```python
from build123d import *

# Parameters (mm, degrees)
F0_R     = 15.054767
F0_R_2   = 12.024096
F1_DEPTH = 100
F2_R     = 14.954944
F2_R_2   = 9.478125
F3_DEPTH = 15.1
F4_DEPTH = 88.3


with BuildPart() as f1:
    # F0 (on Front) → F1 (new body)
    with BuildSketch(Plane.XZ):
        Circle(F0_R)
        Circle(F0_R_2, mode=Mode.SUBTRACT)
    extrude(amount=F1_DEPTH)

    # F2 (on Right) → F3 (join)
    with BuildSketch(Plane.YZ):
        Circle(F2_R)
        Circle(F2_R_2, mode=Mode.SUBTRACT)
    extrude(amount=F3_DEPTH)

    # F2 (on Right) → F4 (join)
    with BuildSketch(Plane.YZ):
        Circle(F2_R)
        Circle(F2_R_2, mode=Mode.SUBTRACT)
    extrude(amount=-F4_DEPTH)


solid = f1.part
```
CAD build for the part. Positions are in the model's coordinates, mm. A direction names the side the tool comes from. Round coordinates to 2 decimals unless told otherwise and drop trailing zeros. Loops run counter-clockwise (first coordinate to the right, second up) from the corner with the lowest first, then second, coordinate; pieces in that order, holes last. Notation, with made-up numbers: M -34,41.25 L 9,41.25 A34 ccw 9,71.25 Z; hole C 44.5,54 d2. An arc over 180 degrees is marked long. Return JSON: item names as keys, results as strings. Group by question number.
(1) Saw through at B-B, the plane x = 9. List the corners of the cut face in (y, z), and give its area (3 significant figures).
(2) Saw through at C-C, the plane y = -90. List the corners of the cut face in (x, z).
(3) Mould opens along Y. For faces 1 (the cylindrical face through (15.054, -3.62, -0.144)), 2 (the flat face through (-10, -100, -7)), 3 (the cylindrical face through (-15.04, -49.3, 0.66)) say: +Y half, -Y half, draft (parallel to the pull), parting line (faces both ways), or undercut.
(4) Wall check: probe 1 along Y at (x, z) = (-22, 0); probe 2 along X at (y, z) = (-45, 0). Give the ranges that are in metal, low to high. Write a range as [from, to].
(5) Tool access for faces 4 (the cylindrical face through (-12.012, -53.808, 0.529)), 5 (the flat face through (15.1, 0, -10)), 6 (the cylindrical face through (12.023, -3.62, -0.153)), 7 (the flat face through (-88.3, 0, -10)), 8 (the flat face through (-13, 0, 0)): list every direction of +Z, -Z, +X, -X, +Y, -Y with a clear straight run to the whole face (end or side of a thin tool).
(6) Saw through at D-D, the plane x = -41.5. List the corners of the cut face in (y, z).
(7) Saw through at A-A, the plane z = 0. List the corners of the cut face in (x, y).
(8) Drop flat-ended pins along their axis: P1, Ø12, axis at x = -44, y = -4.5, coming from the +Z side; P2, Ø5, axis at y = -27.5, z = 4, coming from the +X side; P3, Ø2.5, axis at x = -12, z = 1, coming from the +Y side; P4, Ø8, axis at x = 3.5, z = 10, coming from the +Y side. Give the stop position or say it passes through.
Answer list:
{
 "1": {"outline": "M -100,-12.07 L -8.83,-12.07 A14.95 ccw long -8.83,12.07 L -100,12.07 L -100,7.97 L -12.65,7.97 A14.95 ccw -12.65,-7.97 L -100,-7.97 Z; hole M -5.12,-7.97 L 0,-7.97 L 0,-9.48 A9.48 ccw 0,9.48 L 0,7.97 L -5.12,7.97 A9.48 ccw Z", "area": "1,160 mm2"},
 "2": {"outline": "C 0,0 d30.11; hole C 0,0 d24.05"},
 "3": {"face 1": "undercut", "face 2": "-Y half", "face 3": "draft"},
 "4": {"probe 1": "[-14.95, -9.48], [9.48, 14.95]", "probe 2": "[-15.05, -12.02], [12.02, 15.05]"},
 "5": {"face 4": "-Y", "face 5": "+Z, -Z, +X, +Y, -Y", "face 6": "none", "face 7": "+Z, -Z, -X, +Y, -Y", "face 8": "+X, -X"},
 "6": {"outline": "C 0,0 d29.91; hole C 0,0 d18.96"},
 "7": {"outline": "M -88.3,-14.95 L -15.05,-14.95 L -15.05,-100 L -12.02,-100 L -12.02,-14.95 L 12.02,-14.95 L 12.02,-100 L 15.05,-100 L 15.05,-14.95 L 15.1,-14.95 L 15.1,-9.48 L 15.05,-9.48 L 15.05,0 L 12.02,0 L 12.02,-9.48 L -12.02,-9.48 L -12.02,0 L -15.05,0 L -15.05,-9.48 L -88.3,-9.48 Z; M -88.3,9.48 L 15.1,9.48 L 15.1,14.95 L -88.3,14.95 Z"},
 "8": {"P1": "z = 14.95", "P2": "x = 14.98", "P3": "y = 14.95", "P4": "y = 13.7"}
}
